Autodesk Fusion 360 part; units mm, degrees
sketch "Sketch1" plane through (0, 0, 0) normal (0, 0, 1) x (1, 0, 0)
  circle A0 centre (0, 75) radius 1.375
  circle A1 centre (0, 75) radius 2.25
  line L0 (0, 72.75) -> (0, -5)
  circle A2 centre (0, -5) radius 2.5
  line L1 (0, -5) -> (0, -7.5)
  line L2 (1.25, 73.1292) -> (1.25, -2.8349)
  line L3 (-1.25, 73.1292) -> (-1.25, -2.8349)
  dimension "d1" = 2.75
  dimension "d2" = 4.5
  dimension "d3" = 80
  dimension "d4" = 5
revolve "Revolve1" add sketch "Sketch1" angle 360 about axis through (0, -5, 0) along (0, -1, 0) contours L0 A2 L1 picked at (1.6574, -4.8758)
revolve "Revolve2" add sketch "Sketch1" angle 360 about axis through (0, 72.75, 0) along (0, -1, 0) contours A1 L0 A2 L3
extrude "Extrude1" add sketch "Sketch1" along normal mid plane 3 contours A1
chamfer "Chamfer1" distance 0.2 angle 45 2 edges at (-2.0977, 74.1864, 1.5) (-2.0977, 75.8136, -1.5)
CAD build for the part. Positions are in the model's coordinates, mm. A direction names the side the tool comes from. Round coordinates to 2 decimals unless told otherwise and drop trailing zeros. Order: outer loops, then holes, each group sorted by start corner. A loop starts at its lowest first (then second) coordinate and runs counter-clockwise, first axis right, second up. Notation, with made-up numbers: (-31.5, -37) -> (-5.5, -37) arc R24 ccw to (-5.5, -4) -> close; hole circle Ø11 at (-21.5, -36.75). An arc over 180 degrees is marked (long way). One line per question, with ' | ' between items.
Q1. Slice it at B-B (x = 0). Write the cut outline in (y, z) (3 decimals), then the cut area to 3 significant figures.
Completed:
outline: (-2.835, -1.25) -> (72.75, -1.25) -> (72.75, -1.3) -> (72.95, -1.5) -> (73.625, -1.5) -> (73.625, 1.5) -> (72.95, 1.5) -> (72.75, 1.3) -> (72.75, 1.25) -> (-2.835, 1.25) arc R2.5 ccw (long way) to start; (76.375, -1.5) -> (77.05, -1.5) -> (77.25, -1.3) -> (77.25, 1.3) -> (77.05, 1.5) -> (76.375, 1.5) -> close | area: 213 mm^2
Q2. Slice it at C-C (y = 25). Write the cut outline in (x, z).
Completed:
outline: circle Ø2.5 at (0, 0)
Q3. Slice it at A-A (y = 75). Write the cut outline in (x, z) (3 decimals).
Completed:
outline: (-2.25, -1.3) -> (-2.05, -1.5) -> (-1.375, -1.5) -> (-1.375, 1.5) -> (-2.05, 1.5) -> (-2.25, 1.3) -> close; (1.375, -1.5) -> (2.05, -1.5) -> (2.25, -1.3) -> (2.25, 1.3) -> (2.05, 1.5) -> (1.375, 1.5) -> close
Q4. Drop flat-ended pins along their axis: pin 1 (1 mm diameter, centred on x = 0, z = 1, fed in from -Y); pin 2 (1.5 mm diameter, centred on y = 66.5, z = 1.5, fed in from +X); pin 3 (2 mm diameter, centred on x = 0.5, y = 75.5, fed in from -Z). Give the stop position or say it passes through.
Completed:
pin 1: stops at y = -7.45 | pin 2: stops at x = 1 | pin 3: stops at z = -1.5
Q5. Probe probe 1 along X at (y, z) = (75, 0.55) (3 decimals); probe 2 along Y at (x, z) = (0, -0.1) (3 decimals); probe 3 along Y at (x, z) = (0, 0.85) (3 decimals). List the from-to ranges inside material, lowest first.
Completed:
probe 1: x = -2.25 to -1.375, 1.375 to 2.25 | probe 2: y = -7.498 to 73.625, 76.375 to 77.25 | probe 3: y = -7.351 to 73.625, 76.375 to 77.25
Q6. Which spindle directions (+Z, -Z, +X, -X, +Y, -Y) get a long thin tool onto all of the face, cutting with end or side? Do faces 1 (the cylindrical face through (-0.3, 76.34, -0.02)), 2 (the cylindrical face through (-1.19, 34.62, -0.38)). Say none if no direction does.
Completed:
face 1: +Z, -Z | face 2: none
